Model file for the job. Use its own axes, mm. A direction names the side the tool comes from. Give positions to 0.01 mm unless a question says otherwise; leave off trailing zeros. Write each loop counter-clockwise with the first axis right and the second up, starting at its lowest first coordinate (ties: lowest second). Pieces come first, ordered by that corner, then holes.
Autodesk Inventor part; units mm, degrees
ref_plane "YZ Plane" through (0, 0, 0) normal (1, 0, 0) x (0, 1, 0)
ref_plane "XZ Plane" through (0, 0, 0) normal (0, 1, 0) x (-1, 0, 0)
ref_plane "XY Plane" through (0, 0, 0) normal (0, 0, 1) x (1, 0, 0)
sketch "Sketch1" plane through (0, 0, 0) normal (0, 0, 1) x (1, 0, 0)
  line L0 (-4, 25) -> (4, 25)
  line L1 (4, 25) -> (4, -25)
  line L2 (4, -25) -> (-4, -25)
  line L3 (-4, -25) -> (-4, 25)
  circle A0 centre (12.5, 0) radius 2
  circle A1 centre (-12.5, 0) radius 2
  circle A2 centre (21, 0) radius 1.6
  circle A3 centre (0, 21) radius 1.6
  circle A4 centre (-21, 0) radius 1.6
  circle A5 centre (0, -21) radius 1.6
  line L4 (-25, -4) -> (-25, 4)
  line L5 (-25, 4) -> (25, 4)
  line L6 (25, -4) -> (-25, -4)
  line L7 (25, 4) -> (25, -4)
  circle A6 centre (0, 21) radius 4
  circle A7 centre (21, 0) radius 4
  circle A8 centre (-21, 0) radius 4
  circle A9 centre (0, -21) radius 4
  circle A10 centre (12.5, 12.5) radius 8.5
  circle A11 centre (-12.5, 12.5) radius 8.5
  circle A12 centre (-12.5, -12.5) radius 8.5
  circle A13 centre (12.5, -12.5) radius 8.5
  circle A14 centre (0, 0) radius 4
  circle A15 centre (0, 9.5) radius 2
  circle A16 centre (0, -9.5) radius 2
  point P0 (4, 0)
  point P1 (0, 25)
  point P2 (-25, 0)
  point P3 (0, 4)
  point P4 (12.5, 4)
  point P5 (4, 12.5)
  point P6 (4, 21)
  point P7 (-4, 21)
  point P8 (-4, 12.5)
  point P9 (-12.5, 4)
  point P10 (-21, 4)
  point P11 (-21, -4)
  point P12 (-12.5, -4)
  point P13 (-4, -12.5)
  point P14 (-4, -21)
  point P15 (4, -21)
  point P16 (4, -12.5)
  point P17 (12.5, -4)
  point P18 (21, -4)
  point P19 (21, 4)
  point P20 (4, 4)
  point P21 (4, -4)
  point P22 (-4, -4)
  point P23 (-4, 4)
  point P24 (0, 4)
  point P25 (0, -4)
  point P26 (-4, 0)
  dimension "d0" = 4
  dimension "d3" = 360
  dimension "d5" = 3.2
  dimension "d8" = 360
  dimension "d10" = 8
  dimension "d13" = 90
  dimension "d15" = 50
  dimension "d16" = 42
  dimension "d17" = 4
  dimension "d19" = 17
  dimension "d22" = 360
  dimension "d27" = 4
  dimension "d30" = 360
  dimension "d32" = 19
  dimension "d33" = 25
extrude "Extrusion1" add sketch "Sketch1" along normal blind 3 contours A6 | A6 L1 L5 L3 | L3 L5 A11 | A10 L5 L1 | L5 A14 L3 | L3 L6 A8 L5 | L5 A7 L6 L1 | L1 A14 L5 | A14 L6 L3 | A8 | L1 L6 A14 | A7 | L6 L1 A9 L3 | L3 A12 L6 | L6 A13 L1 | A9
properties part number "ACOPLE"
1. Slice it at C-C, the plane y = 0. Write the cut outline in (x, z), and give its area (3 significant figures).
Calculated:
outline: (-25, 0) - (-22.6, 0) - (-22.6, 3) - (-25, 3) - close; (-19.4, 0) - (-14.5, 0) - (-14.5, 3) - (-19.4, 3) - close; (-10.5, 0) - (-4, 0) - (-4, 3) - (-10.5, 3) - close; (4, 0) - (10.5, 0) - (10.5, 3) - (4, 3) - close; (14.5, 0) - (19.4, 0) - (19.4, 3) - (14.5, 3) - close; (22.6, 0) - (25, 0) - (25, 3) - (22.6, 3) - close
area: 82.8 mm2
2. Pin check, flat tips, straight feed: P1, Ø1.5, axis at y = 15, z = 1.5, coming from the +X side; P2, Ø0.9, axis at y = 17.5, z = 1.5, coming from the -X side; P3, Ø1.5, axis at x = 14.5, z = 1.5, coming from the +Y side. Stop position of each tip, or through.
Calculated:
P1: stops at x = 4
P2: stops at x = -4
P3: stops at y = 4
3. Slice it at B-B, the plane z = 0.65. State how many separate pieces and enclosed holes the cut face has, and give its area (3 significant figures).
Calculated:
separate pieces: 1
enclosed holes: 9
area: 638 mm2
4. Probe probe 1 along Y at (x, z) = (0, 1.55); probe 2 along Y at (x, z) = (-21, 1.15); probe 3 along Y at (x, z) = (16, 1). List the from-to ranges inside material, lowest first.
Calculated:
probe 1: y = -25 to -22.6, -19.4 to -11.5, -7.5 to -4, 4 to 7.5, 11.5 to 19.4, 22.6 to 25
probe 2: y = -4 to -1.6, 1.6 to 4
probe 3: y = -4 to 4
5. Pull direction Y, two halves, no side cores. Call faces 4 (the flat face through (-4, -17, 1)), 5 (the flat face through (-17, -4, 1)), 6 (the cylindrical face through (0, 25, 1)), 7 (the cylindrical face through (-0.208, -22.586, 1.479)): +Y half, -Y half, draft (parallel to the pull), parting line (faces both ways), or undercut.
Calculated:
face 4: draft
face 5: -Y half
face 6: +Y half
face 7: undercut
6. Slice it at D-D, the plane x = 11.5. Write the cut outline in (y, z).
Calculated:
outline: (-4.06, 0) - (-1.73, 0) - (-1.73, 3) - (-4.06, 3) - close; (1.73, 0) - (4.06, 0) - (4.06, 3) - (1.73, 3) - close
7. Which spindle directions (+Z, -Z, +X, -X, +Y, -Y) get a long thin tool onto all of the face, cutting with end or side? Do faces 1 (the flat face through (-2, -4, 0)), 2 (the flat face through (-17, 4, 1)), 3 (the flat face through (4, 17, 1)). Say none if no direction does.
Calculated:
face 1: -Z, +X, -X, +Y, -Y
face 2: +Z, -Z, -X, +Y
face 3: +Z, -Z, +X, +Y
8. Slice it at A-A, the plane x = 0. Write the cut outline in (y, z).
Calculated:
outline: (-25, 0) - (-22.6, 0) - (-22.6, 3) - (-25, 3) - close; (-19.4, 0) - (-11.5, 0) - (-11.5, 3) - (-19.4, 3) - close; (-7.5, 0) - (-4, 0) - (-4, 3) - (-7.5, 3) - close; (4, 0) - (7.5, 0) - (7.5, 3) - (4, 3) - close; (11.5, 0) - (19.4, 0) - (19.4, 3) - (11.5, 3) - close; (22.6, 0) - (25, 0) - (25, 3) - (22.6, 3) - close
